Could you check a few things on this model? Use its own coordinates, in mm. A direction names the side the tool comes from. Give positions to 0.01 mm unless a question says otherwise; leave off trailing zeros. Loops run counter-clockwise (first coordinate to the right, second up) from the corner with the lowest first, then second, coordinate; pieces in that order, holes last. Notation, with made-up numbers: (29, -29) - (49, -29) arc R20 ccw to (49, -4) - close; hole circle Ø7 at (76.25, 44). An arc over 180 degrees is marked (long way). Write each question's results on one line, items separated by ' | '. Start each with the question number.
(1) Suppose I cut it at C-C (y = 77). Please give me the cut outline in (x, z).
(2) If we mould it in two halves opening along X, with no side actions, what happens to faces 6 (the face through (-116.216, 69, 31)), 7 (the face through (52.12, 28.42, 30.55)), 8 (the face through (-100, 7.049, 31)), 9 (the face through (-43, 33.517, 31))? For each: released by +X, released by -X, zero draft, split by the parting line, or undercut.
(3) Suppose I cut it at D-D (x = -72). Please give me the cut outline in (y, z).
(4) Suppose I cut it at A-A (z = 10). Please give me the cut outline in (x, y).
(5) For pin 1 (1.5 mm diameter, centred on x = 14.5, z = 9, fed in from -Y); pin 2 (4 mm diameter, centred on y = -4, z = 16.5, fed in from +X); pin 3 (10.5 mm diameter, centred on x = -40.5, z = 39, fed in from +Y), each with a flat end and sliding along its axis, tell me the tip position at first contact or that it passes through.
(6) I need wall thicknesses on line 1 (Y direction, x = -98.5, z = 47); line 2 (X direction, y = 113, z = 28); line 3 (X direction, y = 74.5, z = 9). Which ranges of each line are inside material? Lowest first, please.
(7) On a 3-axis mill with a long thin cutter (end or side, diameter ignored), from which of +Z, -Z, +X, -X, +Y, -Y can I reach the whole of each face in a straight line? I mean faces 1 (the face through (-35.884, -7, 31)), 2 (the face through (-60, -13.946, 31)), 3 (the face through (-24, 74.726, 31)), 4 (the face through (-36.042, 20, 31)), 5 (the face through (-48, 46, 0)). Say none if no direction works.
(8) Suppose I cut it at B-B (x = -43.5). Please give me the cut outline in (y, z), and give its area (3 significant figures).
from build123d import *

# Parameters (mm, degrees)
F0_W     = 13.1786922227
F0_H     = 41.2089657038
F0_W_2   = 66.9952295721
F0_H_2   = 54.149620235
F0_W_3   = 34.1263301671
F0_H_3   = 26.4682687528
F1_DEPTH = 61.976


with BuildPart() as f1:
    # F0 (on Top) → F1 (new body)
    with BuildSketch(Plane.XY):
        Polygon((-49.2211245, 0), (-35.8841195703, 0), (-35.8841195703, 33.5169229656), (-36.0424322773, 33.5169229656), (-36.0424322773, 7.0486542129), (-49.2211245, 7.0486542129), align=None)
        Polygon((-31.6636036608, 30.3650720171), (-31.5128481644, 0), (0, 0), (0, 55.8741530566), align=None)
        with Locations((-42.6317783887, 54.1214058176)):
            Rectangle(F0_W, F0_H)
        Polygon((0, 0), (-31.5128481644, 0), (-31.4532000547, -12.0142826496), (1.8114981332, -38.2728779304), (43.0814946911, -28.637456001), (61.2796404565, 9.6363138989), (42.7023604934, 47.7275023921), (1.3387255216, 56.9526676245), (0, 55.8741530566), align=None)
        Polygon((-116.2163540721, 7.0486542129), (-83.3474546671, 7.0486542129), (-83.3474546671, 33.5169229656), (-49.2211245, 33.5169229656), (-49.2211245, 74.7258886695), (-116.2163540721, 74.7258886695), align=None)
        with Locations((-82.7187392861, 101.800698787)):
            Rectangle(F0_W_2, F0_H_2)
        with Locations((-66.2842895836, 20.2827885893)):
            Rectangle(F0_W_3, F0_H_3)
        Polygon((-35.8841195703, 33.5169229656), (-35.8841195703, 0), (-31.5128481644, 0), (-31.6636036608, 30.3650720171), (0, 55.8741530566), (0, 74.7258886695), (-36.0424322773, 74.7258886695), (-36.0424322773, 33.5169229656), align=None)
        Polygon((-83.3474546671, -13.9464121312), (-35.8841195703, -13.9464121312), (-35.8841195703, 0), (-49.2211245, 0), (-49.2211245, 7.0486542129), (-83.3474546671, 7.0486542129), align=None)
    extrude(amount=F1_DEPTH)


solid = f1.part
Output values:
1) outline: (-116.22, 0) - (-49.22, 0) - (-49.22, 61.98) - (-116.22, 61.98) - close
2) face 6: released by -X | face 7: released by +X | face 8: zero draft | face 9: undercut
3) outline: (-13.95, 0) - (128.88, 0) - (128.88, 61.98) - (-13.95, 61.98) - close
4) outline: (-116.22, 7.05) - (-83.35, 7.05) - (-83.35, -13.95) - (-35.88, -13.95) - (-35.88, 0) - (-31.51, 0) - (-31.45, -12.01) - (1.81, -38.27) - (43.08, -28.64) - (61.28, 9.64) - (42.7, 47.73) - (1.34, 56.95) - (0, 55.87) - (0, 74.73) - (-49.22, 74.73) - (-49.22, 128.88) - (-116.22, 128.88) - close; hole (-49.22, 7.05) - (-36.04, 7.05) - (-36.04, 33.52) - (-49.22, 33.52) - close
5) pin 1: y = -35.49 | pin 2: x = 55.75 | pin 3: y = 74.73
6) line 1: 7.05 to 128.88 | line 2: -116.22 to -49.22 | line 3: -116.22 to 0
7) face 1: +Z, -Z, -Y | face 2: +Z, -Z, -X, -Y | face 3: +Z, -Z, +X, +Y | face 4: +Z, -Z | face 5: -Z, +X, -X, +Y, -Y
8) outline: (-13.95, 0) - (7.05, 0) - (7.05, 61.98) - (-13.95, 61.98) - close; (33.52, 0) - (74.73, 0) - (74.73, 61.98) - (33.52, 61.98) - close | area: 3,860 mm2
